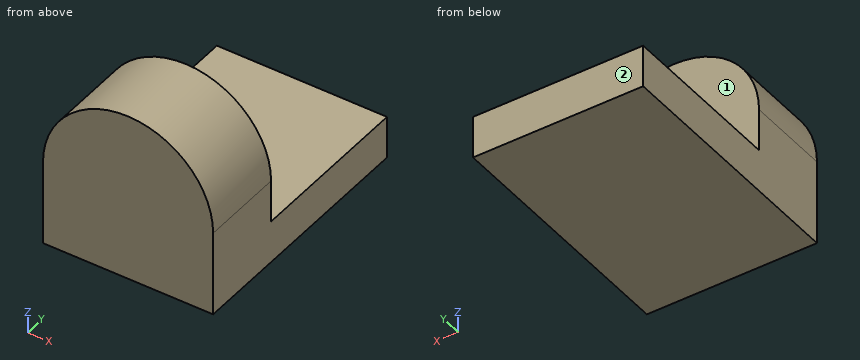
```python
from build123d import *

# Parameters (mm, degrees)
F1_DEPTH = 38.1
F3_DEPTH = 25.4


with BuildPart() as f1:
    # F0 (on Front) → F1 (new body)
    with BuildSketch(Plane.XZ):
        with BuildLine():
            Line((0, 12.7), (0, 0))
            Line((0, 0), (25.4, 0))
            Line((25.4, 0), (25.4, 12.7))
            ThreePointArc((25.4, 12.7), (12.7, 25.4), (0, 12.7))
        make_face()
    extrude(amount=F1_DEPTH)

    # F2 (on Front) → F3 (cut)
    with BuildSketch(Plane.XZ):
        with BuildLine():
            Line((0, 12.7), (0, 6.35))
            Line((0, 6.35), (25.4, 6.35))
            Line((25.4, 6.35), (25.4, 12.7))
            ThreePointArc((25.4, 12.7), (12.7, 25.4), (0, 12.7))
        make_face()
    extrude(amount=F3_DEPTH, mode=Mode.SUBTRACT)


solid = f1.part
```
Part model, mm, in its own coordinate system. Face numbers are marked on the shaded views. A direction names the side the tool comes from. Round coordinates to 2 decimals unless told otherwise and drop trailing zeros. Order: outer loops, then holes, each group sorted by start corner. A loop starts at its lowest first (then second) coordinate and runs counter-clockwise, first axis right, second up. Notation, with made-up numbers: M 7.5,2.25 L 45.5,2.25 A19 cw 45.5,29.25 Z; hole C -24,65 d6. An arc over 180 degrees is marked long. Answer in a Markdown table with one row per item. Add a question column.
Q1. Cut at A-A on x = 12.7. Give the cut face in (y, z).
Q2. Cut at D-D on x = 22.5. Give the cut face in (y, z), and give its area (3 significant figures).
Q3. Pin check, flat tips, straight feed: pin 1 (4 mm diameter, centred on y = -23.5, z = 7, fed in from -X); pin 2 (5.5 mm diameter, centred on x = 13.5, z = 15.5, fed in from +Y); pin 3 (12 mm diameter, centred on y = -23.5, z = 21.5, fed in from -X); pin 4 (10 mm diameter, centred on y = -29.5, z = 20, fed in from -X). Stop position of each tip, or through.
Q4. Cut at C-C on z = 9.75. Give the cut face in (x, y), and give its area (3 significant figures).
Q5. 3-axis set-ups, long thin cutter, end or side, ignore diameter. For the marked faces 1 and 2: which of +Z, -Z, +X, -X, +Y, -Y reach the whole face in a straight line?
Q6. Cut at B-B on y = -35. Give the cut face in (x, z).
Q7. Wall check: L1, parallel to Z at x = 23, y = -6; L2, parallel to Y at x = 23.5, z = 16.25; L3, parallel to Z at x = 19.25, y = -29. Give the ranges that are in metal, low to high. Write a range as from..to.
Established:
| question | item | result |
|---|---|---|
| 1 | outline | M -38.1,0 L 0,0 L 0,6.35 L -25.4,6.35 L -25.4,25.4 L -38.1,25.4 Z |
| 2 | outline | M -38.1,0 L 0,0 L 0,6.35 L -25.4,6.35 L -25.4,20.78 L -38.1,20.78 Z |
| 2 | area | 425 mm2 |
| 3 | pin 1 | stops at x = 0 |
| 3 | pin 2 | stops at y = -25.4 |
| 3 | pin 3 | stops at x = 0.39 |
| 3 | pin 4 | stops at x = 0.21 |
| 4 | outline | M 0,-38.1 L 25.4,-38.1 L 25.4,-25.4 L 0,-25.4 Z |
| 4 | area | 323 mm2 |
| 5 | face 1 | +Z, +X, -X, +Y |
| 5 | face 2 | +Z, -Z, +X, -X, +Y |
| 6 | outline | M 0,0 L 25.4,0 L 25.4,12.7 A12.7 ccw 0,12.7 Z |
| 7 | L1 | z = 0..6.35 |
| 7 | L2 | y = -38.1..-25.4 |
| 7 | L3 | z = 0..23.58 |
